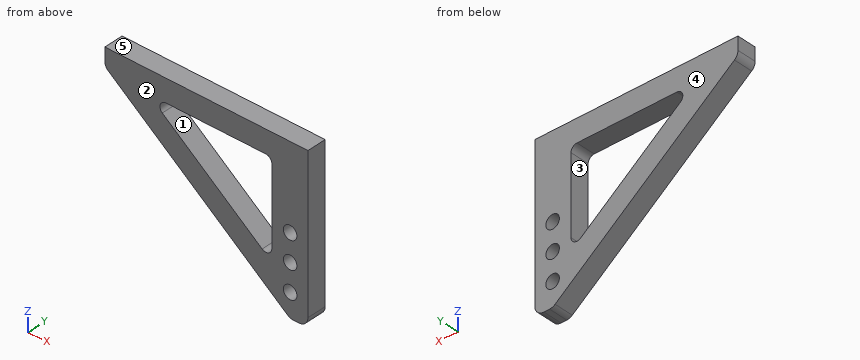
```python
from build123d import *

# Parameters (mm, degrees)
SKETCH1_R           = 0.5715
BOSS_EXTRUDE1_DEPTH = 1.6256
FILLET1_R           = 0.508
FILLET2_R           = 0.762


with BuildPart() as part:
    # Sketch1 → Boss-Extrude1 (new body)
    with BuildSketch(Plane(origin=(0, 0, 0), x_dir=(1, 0, 0), z_dir=(0, 1, 0))):
        Polygon((1.905, 1.4732), (17.54785055, 13.570337759), (19.05, 13.570337759), (19.05, 0), (1.905, 0), align=None)
        with Locations(Location((17.54785055, 11.562216741, 0), (0, 0, 270))):
            Circle(SKETCH1_R, mode=Mode.SUBTRACT)
        with Locations(Location((17.54785055, 9.276216741, 0), (0, 0, 270))):
            Circle(SKETCH1_R, mode=Mode.SUBTRACT)
        with Locations(Location((17.54785055, 6.990216741, 0), (0, 0, 270))):
            Circle(SKETCH1_R, mode=Mode.SUBTRACT)
        Polygon((5.577391241, 1.905), (16.002, 1.905), (16.002, 9.96669744), align=None, mode=Mode.SUBTRACT)
    extrude(amount=BOSS_EXTRUDE1_DEPTH)

    # Fillet1
    fillet1_edges = [part.edges().sort_by_distance(p)[0] for p in [
        (16.002, 0.8128, -9.96669744),
        (5.577391241, 0.8128, -1.905),
        (16.002, 0.8128, -1.905),
    ]]
    fillet(fillet1_edges, radius=FILLET1_R)

    # Fillet2
    fillet2_edges = [part.edges().sort_by_distance(p)[0] for p in [
        (1.905, 0.8128, -1.4732),
        (17.54785055, 0.8128, -13.570337759),
        (19.05, 0.8128, -13.570337759),
    ]]
    fillet(fillet2_edges, radius=FILLET2_R)


solid = part.part
```
Could you check a few things on this model? Use its own coordinates, in mm. Face numbers are marked on the shaded views. A direction names the side the tool comes from. Give positions to 0.01 mm unless a question says otherwise; leave off trailing zeros. Write each loop counter-clockwise with the first axis right and the second up, starting at its lowest first coordinate (ties: lowest second). Pieces come first, ordered by that corner, then holes. Notation, with made-up numbers: (13.5, -5.5) - (59.5, -5.5) arc R9 cw to (59.5, 2.5) - close; hole circle Ø7 at (76.25, -3). An arc over 180 degrees is marked (long way). One line per item, written item: value. Start each with the question number.
Item 1: Imagine slicing it at C-C, the plane y = 1.1. Give the number of separate pieces and of enclosed holes in the cut face, and give its area (3 significant figures).
Item 2: Imagine slicing it at A-A, the plane z = -3.75. List the corners of the cut face in (x, y) for me, and give its area (3 significant figures).
Item 3: Please list where these lines run through material, in increasing order: line 1 (Z direction, x = 18, y = 0.15); line 2 (Z direction, x = 17.25, y = 1.55); line 3 (Z direction, x = 12.5, y = 1.55) (3 decimals). Write a range as from..to.
Item 4: I'm going to push flat-ended pins straight in: pin 1 (0.5 mm diameter, centred on y = 0.5, z = -5.5, fed in from -X); pin 2 (0.5 mm diameter, centred on x = 12, y = 1, fed in from -Z). Where does each tip first touch, or does it pass through?
Item 5: Imagine slicing it at B-B, the plane x = 15.75. List the corners of the cut face in (y, z) for me.
Item 6: Imagine slicing it at D-D, the plane x = 4.5. List the corners of the cut face in (y, z) for me, and give its area (3 significant figures).
Item 7: Which directions (+Z, -Z, +X, -X, +Y, -Y) give clear straight access to the entire face, cutting with the end or side of a thin tool? Please do the marked faces 1 and 2.
Item 8: If we mould it in two halves opening along Z, with no side actions, what happens to the marked faces 3, 4 and 5? For each: +Z half, -Z half, draft (parallel to the pull), parting line (faces both ways), or undercut.
Geometry says:
1. separate pieces: 1
1. enclosed holes: 4
1. area: 93.5 mm^2
2. outline: (4.85, 0) - (7.96, 0) - (7.96, 1.63) - (4.85, 1.63) - close; (16, 0) - (19.05, 0) - (19.05, 1.63) - (16, 1.63) - close
2. area: 10.0 mm^2
3. line 1: -13.57..-11.91, -11.21..-9.63, -8.93..-7.34, -6.64..0
3. line 2: -13.34..-12.05, -11.07..-9.76, -8.79..-7.48, -6.5..0
3. line 3: -9.667..-7.258, -1.905..0
4. pin 1: x = 6.79
4. pin 2: z = -9.47
5. outline: (0, -12.18) - (1.63, -12.18) - (1.63, -9.37) - (0, -9.37) - close; (0, -1.97) - (1.63, -1.97) - (1.63, 0) - (0, 0) - close
6. outline: (0, -3.48) - (1.63, -3.48) - (1.63, 0) - (0, 0) - close
6. area: 5.66 mm^2
7. face 1: +Y, -Y
7. face 2: +Z, -Z, +X, -X, -Y
8. face 3: undercut
8. face 4: draft
8. face 5: +Z half
